The model under review builds one solid part; all positions refer to its coordinate system, in mm. A direction names the side the tool comes from. Round coordinates to 2 decimals unless told otherwise and drop trailing zeros. Write each loop counter-clockwise with the first axis right and the second up, starting at its lowest first coordinate (ties: lowest second). Pieces come first, ordered by that corner, then holes. Notation, with made-up numbers: (25.25, 46) - (49.25, 46) arc R17 cw to (49.25, 79) - close; hole circle Ø1 at (7, 38.25). An arc over 180 degrees is marked (long way). Use one line per item in the form item = value.
from build123d import *
from OCP.BRepFilletAPI import BRepFilletAPI_MakeChamfer

# Parameters (mm, degrees)
SKETCH_1_R          = 2.85
EXTRUDE_1_DEPTH     = 1.4
FILLET_1_R          = 1.4
SKETCH_3_R          = 1.5
EXTRUDE_3_DEPTH     = 6
CUT_EXTRUDE_1_DEPTH = 1
CHAMFER_2_SIZE      = 0.3
CHAMFER_3_SIZE      = 0.576368876
CHAMFER_3_SIZE2     = 0.998300177
FILLET_2_R          = 0.1


with BuildPart() as part:
    # 草图1 → 凸台-拉伸1 (new body)
    with BuildSketch(Plane.XY):
        Circle(SKETCH_1_R)
    extrude(amount=EXTRUDE_1_DEPTH)

    # 圆角1
    fillet_1_edges = [part.edges().sort_by_distance(p)[0] for p in [
        (-2.85, 0, 1.4),
    ]]
    fillet(fillet_1_edges, radius=FILLET_1_R - 0.0001)  # a hair under: the kernel refuses the full size

    # 草图3 → 凸台-拉伸3 (add)
    with BuildSketch(Plane(origin=(0, 0, 0), x_dir=(-1, 0, 0), z_dir=(0, 0, -1))):
        with Locations(Location((0, 0, 0), (0, 0, 180))):
            Circle(SKETCH_3_R)
    extrude(amount=EXTRUDE_3_DEPTH)

    # 草图4 → 切除-拉伸1 (cut)
    with BuildSketch(Plane.XY.offset(1.4)):
        Polygon((1, 0.577350269), (0, 1.154700538), (-1, 0.577350269), (-1, -0.577350269), (0, -1.154700538), (1, -0.577350269), align=None)
    extrude(amount=-CUT_EXTRUDE_1_DEPTH, mode=Mode.SUBTRACT)

    # 倒角2
    chamfer_2_edges = [part.edges().sort_by_distance(p)[0] for p in [
        (-1.5, 0, -6),
    ]]
    chamfer(chamfer_2_edges, length=CHAMFER_2_SIZE)

    # 倒角3: one chamfer whose edges measure the first distance from different faces: ONE call of the kernel's chamfer builder (chamfer() names one face for all edges)
    chamfer_3_edges_1 = [part.edges().sort_by_distance(p)[0] for p in [
        (1, 0, 0.4),
    ]]
    chamfer_3_side_1 = [part.faces().sort_by_distance(p)[0] for p in [
        (1, 0, 0.9),
    ]]
    chamfer_3_edges_2 = [part.edges().sort_by_distance(p)[0] for p in [
        (0.5, -0.866025404, 0.4),
    ]]
    chamfer_3_side_2 = [part.faces().sort_by_distance(p)[0] for p in [
        (0.5, -0.866025404, 0.9),
    ]]
    chamfer_3_edges_3 = [part.edges().sort_by_distance(p)[0] for p in [
        (-0.5, -0.866025404, 0.4),
    ]]
    chamfer_3_side_3 = [part.faces().sort_by_distance(p)[0] for p in [
        (-0.5, -0.866025404, 0.9),
    ]]
    chamfer_3_edges_4 = [part.edges().sort_by_distance(p)[0] for p in [
        (-1, 0, 0.4),
    ]]
    chamfer_3_side_4 = [part.faces().sort_by_distance(p)[0] for p in [
        (-1, 0, 0.9),
    ]]
    chamfer_3_edges_5 = [part.edges().sort_by_distance(p)[0] for p in [
        (-0.5, 0.866025404, 0.4),
    ]]
    chamfer_3_side_5 = [part.faces().sort_by_distance(p)[0] for p in [
        (-0.5, 0.866025404, 0.9),
    ]]
    chamfer_3_edges_6 = [part.edges().sort_by_distance(p)[0] for p in [
        (0.5, 0.866025404, 0.4),
    ]]
    chamfer_3_side_6 = [part.faces().sort_by_distance(p)[0] for p in [
        (0.5, 0.866025404, 0.9),
    ]]
    chamfer_3 = BRepFilletAPI_MakeChamfer(part.part.solid().wrapped)
    for e in chamfer_3_edges_1:
        chamfer_3.Add(CHAMFER_3_SIZE, CHAMFER_3_SIZE2, e.wrapped, chamfer_3_side_1[0].wrapped)  # the first distance lies on this face
    for e in chamfer_3_edges_2:
        chamfer_3.Add(CHAMFER_3_SIZE, CHAMFER_3_SIZE2, e.wrapped, chamfer_3_side_2[0].wrapped)  # the first distance lies on this face
    for e in chamfer_3_edges_3:
        chamfer_3.Add(CHAMFER_3_SIZE, CHAMFER_3_SIZE2, e.wrapped, chamfer_3_side_3[0].wrapped)  # the first distance lies on this face
    for e in chamfer_3_edges_4:
        chamfer_3.Add(CHAMFER_3_SIZE, CHAMFER_3_SIZE2, e.wrapped, chamfer_3_side_4[0].wrapped)  # the first distance lies on this face
    for e in chamfer_3_edges_5:
        chamfer_3.Add(CHAMFER_3_SIZE, CHAMFER_3_SIZE2, e.wrapped, chamfer_3_side_5[0].wrapped)  # the first distance lies on this face
    for e in chamfer_3_edges_6:
        chamfer_3.Add(CHAMFER_3_SIZE, CHAMFER_3_SIZE2, e.wrapped, chamfer_3_side_6[0].wrapped)  # the first distance lies on this face
    add(Compound.cast(chamfer_3.Shape()), mode=Mode.REPLACE)

    # 圆角2
    fillet_2_edges = [part.edges().sort_by_distance(p)[0] for p in [
        (-1.5, 0, 0),
    ]]
    fillet(fillet_2_edges, radius=FILLET_2_R)


solid = part.part
(1) Insertion check: P1, Ø1.5, axis at y = 0.5, z = -2.5, coming from the -X side; P2, Ø1.5, axis at y = 1.5, z = -2, coming from the +X side. Each pin has a flat end and moves straight along its axis. Give the tip position at first contact, or say it passes through.
Geometry results:
P1 = -1.5
P2 = 1.3
(2) To check wall thickness, follow L1, parallel to Y at x = 0.05, z = -4.5; L2, parallel to Y at x = 0.9, z = -0.5; L3, parallel to Y at x = 0.5, z = 1.25. State the ranges of each line that lie inside material, in increasing order.
Geometry results:
L1 = -1.5 to 1.5
L2 = -1.2 to 1.2
L3 = -2.02 to -0.87, 0.87 to 2.02
(3) Machinability: for faces 4 (the flat face through (0, 0, -6)), 5 (the flat face through (0, -2, 0)), 6 (the flat face through (0.3, -0.53, 0.75)), which of the approach directions +Z, -Z, +X, -X, +Y, -Y give a long, thin tool a straight path to every point of the face, cutting with its end or side? Answer none if there is none.
Geometry results:
face_4 = -Z, +X, -X, +Y, -Y
face_5 = -Z
face_6 = +Z
(4) Add section A-A on z = -4.75. Write out the cut boundary in (x, y), then the cut area to 3 significant figures.
Geometry results:
outline = circle Ø3 at (0, 0)
area = 7.07 mm2
(5) The part is to be moulded in two halves that separate along Y. For faces 1 (the cylindrical face through (1.43, -0.45, -2.86)), 2 (the flat face through (0.6, 1, 1.4)), 3 (the flat face through (0.31, 0.52, 0.75)), say which applies: +Y half, -Y half, draft (parallel to the pull), parting line (faces both ways), or undercut.
Geometry results:
face_1 = parting line
face_2 = draft
face_3 = undercut
